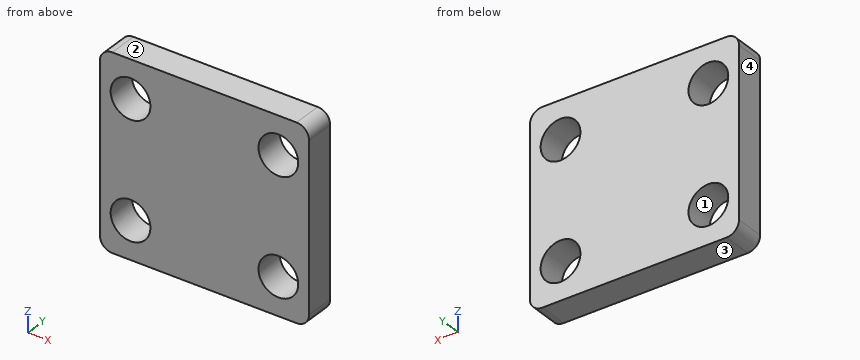
from build123d import *

# Parameters (mm, degrees)
ESQUISSE1_W             = 42.7228
ESQUISSE1_H             = 39.2176
BOSS_EXTRU_1_DEPTH      = 12.573
ENL_V_MAT_EXTRU_1_DEPTH = 40.2176
PER_AGE1_D              = 8.128
PER_AGE1_DEPTH          = 12.573
CONG_1_R                = 0.254
CONG_2_R                = 2.54
ESQUISSE5_W             = 59.007175712
ESQUISSE5_H             = 21.340180089
ENL_V_MAT_EXTRU_2_DEPTH = 43.7228


with BuildPart() as part:
    # Esquisse1 → Boss.-Extru.1 (new body)
    with BuildSketch(Plane(origin=(0, 12.573, 0), x_dir=(1, 0, 0), z_dir=(0, 1, 0))):
        Rectangle(ESQUISSE1_W, ESQUISSE1_H)
    extrude(amount=-BOSS_EXTRU_1_DEPTH)

    # Esquisse2 → Enlèv. mat.-Extru.1 (cut, through all)
    with BuildSketch(Plane(origin=(0, 0, -19.6088), x_dir=(-1, 0, 0), z_dir=(0, 0, -1))):
        Polygon((-9.525, 12.573), (-6.985, 7.493), (6.985, 7.493), (9.525, 12.573), align=None)
    extrude(amount=-ENL_V_MAT_EXTRU_1_DEPTH, mode=Mode.SUBTRACT)

    # Perçage1
    with Locations(Plane(origin=(0, 12.573, 0), x_dir=(1, 0, 0), z_dir=(0, 1, 0))):
        with Locations((15.1003, -11.8745), (-15.1003, 11.8745), (15.1003, 11.8745), (-15.1003, -11.8745)):
            Hole(PER_AGE1_D / 2, depth=PER_AGE1_DEPTH)

    # Congé1
    cong_1_edges = [part.edges().sort_by_distance(p)[0] for p in [
        (9.525, 12.573, 0),
        (-9.525, 12.573, 0),
        (-6.985, 7.493, 0),
        (6.985, 7.493, 0),
    ]]
    fillet(cong_1_edges, radius=CONG_1_R)

    # Congé2
    cong_2_edges = [part.edges().sort_by_distance(p)[0] for p in [
        (21.3614, 6.2865, -19.6088),
        (21.3614, 6.2865, 19.6088),
        (-21.3614, 6.2865, 19.6088),
        (-21.3614, 6.2865, -19.6088),
    ]]
    fillet(cong_2_edges, radius=CONG_2_R)

    # Esquisse5 → Enlèv. mat.-Extru.2 (cut, through all)
    with BuildSketch(Plane(origin=(21.3614, 0, 0), x_dir=(0, 0, -1), z_dir=(1, 0, 0))):
        with Locations((1.148207214, 16.670090045)):
            Rectangle(ESQUISSE5_W, ESQUISSE5_H)
    extrude(amount=-ENL_V_MAT_EXTRU_2_DEPTH, mode=Mode.SUBTRACT)


solid = part.part
The listing builds one solid part. Answer for the finished solid, in the listing's coordinates (mm). Face numbers are marked on the shaded views. Coordinates: 2 decimals unless noted, no trailing zeros. Order: outer loops, then holes, each group sorted by start corner. A loop starts at its lowest first (then second) coordinate and runs counter-clockwise, first axis right, second up. Notation, with made-up numbers: (68.5, 67) -> (113.5, 67) arc R10 ccw to (113.5, 86) -> close; hole circle Ø10 at (-5, 32.25). An arc over 180 degrees is marked (long way). Answer in a Markdown table with one row per item. Add a question column.
Item 1: Find the intervals of material crossed by L1, parallel to Z at x = -13, y = 5.25; L2, parallel to X at y = 4, z = -12.5; L3, parallel to X at y = 1, z = 13, in increasing order. Write a range as from..to.
Item 2: Determine the mould class of the marked faces 1, 2, 3 and 4 for opening direction Z: +Z half, -Z half, draft (parallel to the pull), parting line (faces both ways), or undercut.
Item 3: Find section A-A (z = 10.5). Write down the section's boundary in (x, y).
Item 4: Find section B-B (y = 1.25). Write down the section's boundary in (x, z).
Item 5: Find section C-C (x = -12). Write down the section's boundary in (y, z), then the cut area to 3 significant figures.
Result set:
| question | item | result |
|---|---|---|
| 1 | L1 | z = -19.61..-15.35, -8.4..8.4, 15.35..19.61 |
| 1 | L2 | x = -21.36..-19.12, -11.08..11.08, 19.12..21.36 |
| 1 | L3 | x = -21.36..-19.01, -11.2..11.2, 19.01..21.36 |
| 2 | face 1 | undercut |
| 2 | face 2 | +Z half |
| 2 | face 3 | -Z half |
| 2 | face 4 | draft |
| 3 | outline | (-21.36, 0) -> (-18.92, 0) -> (-18.92, 6) -> (-21.36, 6) -> close; (-11.28, 0) -> (11.28, 0) -> (11.28, 6) -> (-11.28, 6) -> close; (18.92, 0) -> (21.36, 0) -> (21.36, 6) -> (18.92, 6) -> close |
| 4 | outline | (-21.36, -17.07) arc R2.54 ccw to (-18.82, -19.61) -> (18.82, -19.61) arc R2.54 ccw to (21.36, -17.07) -> (21.36, 17.07) arc R2.54 ccw to (18.82, 19.61) -> (-18.82, 19.61) arc R2.54 ccw to (-21.36, 17.07) -> close; hole circle Ø8.13 at (-15.1, -11.87); hole circle Ø8.13 at (-15.1, 11.87); hole circle Ø8.13 at (15.1, -11.87); hole circle Ø8.13 at (15.1, 11.87) |
| 5 | outline | (0, -19.61) -> (6, -19.61) -> (6, -14.5) -> (0, -14.5) -> close; (0, -9.25) -> (6, -9.25) -> (6, 9.25) -> (0, 9.25) -> close; (0, 14.5) -> (6, 14.5) -> (6, 19.61) -> (0, 19.61) -> close |
| 5 | area | 172 mm² |
